Build history of the part. All positions in model axes, mm. Give positions to 0.01 mm unless a question says otherwise; leave off trailing zeros. Order: outer loops, then holes, each group sorted by start corner. A loop starts at its lowest first (then second) coordinate and runs counter-clockwise, first axis right, second up. Notation, with made-up numbers: (83, 82) - (108, 82) arc R31 cw to (108, 118) - close; hole circle Ø10 at (37.5, 5). An arc over 180 degrees is marked (long way). Use a Markdown table: item, result. Add a question column.
(1) Wall check: line 1 (X direction, y = 1.45, z = 47.5); line 2 (X direction, y = 6.85, z = -47.5); line 3 (Z direction, x = -26, y = 7.25) (3 decimals). Give the ranges that are in metal, low to high.
(2) Slice it at B-B (z = 8.5). Write the cut outline in (x, y), then the cut area to 3 significant figures.
(3) Slice it at C-C (y = 3.25). Count the separate pieces of the cut face and the enclosed holes in it, then the cut area to 3 significant figures.
(4) Flat gauge pins, fed straight in: pin 1 (2 mm diameter, centred on x = 72, z = 46.5, fed in from +Y); pin 2 (1.5 mm diameter, centred on x = -44.5, z = -10, fed in from -Y); pin 3 (4 mm diameter, centred on x = 8.5, z = -37.5, fed in from +Y); pin 4 (3 mm diameter, centred on x = -72.28, z = -47.5, fed in from +Y). Where does each tip first touch, or does it go through?
(5) Slice it at A-A (z = -47.5). Write the cut outline in (x, y), then the cut area to 3 significant figures.
from build123d import *

# Parameters (mm, degrees)
BOSS_EXTRUDE1_DEPTH           = 57.5
CUT_EXTRUDE1_DEPTH            = 7
CUT_EXTRUDE4_START            = -7
CUT_EXTRUDE4_DEPTH            = 99.838825225
CBORE_FOR_M3_SHCS1_AT_2_COUNT = 2
CBORE_FOR_M3_SHCS1_AT_2_PITCH = 95
CBORE_FOR_M3_SHCS1_AT_3_COUNT = 2
CBORE_FOR_M3_SHCS1_AT_3_PITCH = 144.569240482
CBORE_FOR_M3_SHCS1_AT_4_COUNT = 2
CBORE_FOR_M3_SHCS1_AT_4_PITCH = 172.989205714
SKETCH14_R                    = 3.25
CUT_EXTRUDE5_DEPTH            = 102.795596501


with BuildPart() as part:
    # Sketch1 → Boss-Extrude1 (new, symmetric)
    with BuildSketch(Plane.XY):
        Polygon((-82.284620241, 0), (82.284620241, 0), (82.284620241, 8), (3.5, 21.891854213), (-3.5, 21.891854213), (-82.284620241, 8), align=None)
    extrude(amount=BOSS_EXTRUDE1_DEPTH, both=True)

    # Sketch2 → Cut-Extrude1 (cut)
    with BuildSketch(Plane(origin=(-3.849265471, 21.830269287, 0), x_dir=(0.9848077530122079, 0.17364817766693139, 0), z_dir=(-0.17364817766693139, 0.9848077530122079, 0))):
        with BuildLine():
            Line((-46.110814579, 26.6), (-36.110814579, 26.6))
            ThreePointArc((-36.110814579, 26.6), (-34.510814579, 25), (-36.110814579, 23.4))
            Line((-36.110814579, 23.4), (-46.110814579, 23.4))
            ThreePointArc((-46.110814579, 23.4), (-47.710814579, 25), (-46.110814579, 26.6))
        make_face()
        with BuildLine():
            Line((-11.110814579, -26.6), (-21.110814579, -26.6))
            ThreePointArc((-21.110814579, -26.6), (-22.710814579, -25), (-21.110814579, -23.4))
            Line((-21.110814579, -23.4), (-11.110814579, -23.4))
            ThreePointArc((-11.110814579, -23.4), (-9.510814579, -25), (-11.110814579, -26.6))
        make_face()
        with BuildLine():
            Line((-11.110814579, 26.6), (-21.110814579, 26.6))
            ThreePointArc((-21.110814579, 26.6), (-22.710814579, 25), (-21.110814579, 23.4))
            Line((-21.110814579, 23.4), (-11.110814579, 23.4))
            ThreePointArc((-11.110814579, 23.4), (-9.510814579, 25), (-11.110814579, 26.6))
        make_face()
        with BuildLine():
            Line((-46.110814579, -26.6), (-36.110814579, -26.6))
            ThreePointArc((-36.110814579, -26.6), (-34.510814579, -25), (-36.110814579, -23.4))
            Line((-36.110814579, -23.4), (-46.110814579, -23.4))
            ThreePointArc((-46.110814579, -23.4), (-47.710814579, -25), (-46.110814579, -26.6))
        make_face()
    cut_extrude1 = extrude(amount=-CUT_EXTRUDE1_DEPTH, mode=Mode.SUBTRACT)

    # Sketch7 → Cut-Extrude4 (cut, through all)
    # profile 1 of 10: a face of its own
    with BuildSketch(Plane(origin=(-3.849265471, 21.830269287, 0), x_dir=(0.9848077530122079, 0.1736481776669313, 0), z_dir=(-0.1736481776669313, 0.9848077530122079, 0)).offset(CUT_EXTRUDE4_START)):
        with BuildLine():
            ThreePointArc((-32.360814579, 22.125), (-30.327882583, 22.967068004), (-29.485814579, 25))
            Line((-29.485814579, 25), (-34.510814579, 25))
            ThreePointArc((-34.510814579, 25), (-34.979443729, 23.86862915), (-36.110814579, 23.4))
            Line((-36.110814579, 23.4), (-41.110814579, 23.4))
            Line((-41.110814579, 23.4), (-41.110814579, 22.125))
            Line((-41.110814579, 22.125), (-32.360814579, 22.125))
        make_face()
    # profile 2 of 10: a face of its own
    with BuildSketch(Plane(origin=(-3.849265471, 21.830269287, 0), x_dir=(0.9848077530122079, 0.1736481776669313, 0), z_dir=(-0.1736481776669313, 0.9848077530122079, 0)).offset(CUT_EXTRUDE4_START)):
        with BuildLine():
            Line((-32.360814579, 27.875), (-49.860814579, 27.875))
            ThreePointArc((-49.860814579, 27.875), (-52.735814579, 25), (-49.860814579, 22.125))
            Line((-49.860814579, 22.125), (-41.110814579, 22.125))
            Line((-41.110814579, 22.125), (-41.110814579, 23.4))
            Line((-41.110814579, 23.4), (-46.110814579, 23.4))
            ThreePointArc((-46.110814579, 23.4), (-47.710814579, 25), (-46.110814579, 26.6))
            Line((-46.110814579, 26.6), (-36.110814579, 26.6))
            ThreePointArc((-36.110814579, 26.6), (-34.979443729, 26.13137085), (-34.510814579, 25))
            Line((-34.510814579, 25), (-29.485814579, 25))
            ThreePointArc((-29.485814579, 25), (-30.327882583, 27.032931996), (-32.360814579, 27.875))
        make_face()
    # profile 3 of 10: a face of its own
    with BuildSketch(Plane(origin=(-3.849265471, 21.830269287, 0), x_dir=(0.9848077530122079, 0.1736481776669313, 0), z_dir=(-0.1736481776669313, 0.9848077530122079, 0)).offset(CUT_EXTRUDE4_START)):
        with BuildLine():
            ThreePointArc((-36.110814579, 23.4), (-34.979443729, 23.86862915), (-34.510814579, 25))
            Line((-34.510814579, 25), (-41.110814579, 25))
            Line((-41.110814579, 25), (-41.110814579, 23.4))
            Line((-41.110814579, 23.4), (-36.110814579, 23.4))
        make_face()
    # profile 4 of 10: a face of its own
    with BuildSketch(Plane(origin=(-3.849265471, 21.830269287, 0), x_dir=(0.9848077530122079, 0.1736481776669313, 0), z_dir=(-0.1736481776669313, 0.9848077530122079, 0)).offset(CUT_EXTRUDE4_START)):
        with BuildLine():
            Line((-41.110814579, 25), (-34.510814579, 25))
            ThreePointArc((-34.510814579, 25), (-34.979443729, 26.13137085), (-36.110814579, 26.6))
            Line((-36.110814579, 26.6), (-46.110814579, 26.6))
            ThreePointArc((-46.110814579, 26.6), (-47.710814579, 25), (-46.110814579, 23.4))
            Line((-46.110814579, 23.4), (-41.110814579, 23.4))
            Line((-41.110814579, 23.4), (-41.110814579, 25))
        make_face()
    # profile 5 of 10: a face of its own
    with BuildSketch(Plane(origin=(-3.849265471, 21.830269287, 0), x_dir=(0.9848077530122079, 0.1736481776669313, 0), z_dir=(-0.1736481776669313, 0.9848077530122079, 0)).offset(CUT_EXTRUDE4_START)):
        with BuildLine():
            ThreePointArc((-24.860814579, 22.125), (-27.735814579, 25), (-24.860814579, 27.875))
            Line((-24.860814579, 27.875), (-7.360814579, 27.875))
            ThreePointArc((-7.360814579, 27.875), (-4.485814579, 25), (-7.360814579, 22.125))
            Line((-7.360814579, 22.125), (-24.860814579, 22.125))
        make_face()
        with BuildLine():
            ThreePointArc((-11.110814579, 26.6), (-9.510814579, 25), (-11.110814579, 23.4))
            Line((-11.110814579, 23.4), (-21.110814579, 23.4))
            ThreePointArc((-21.110814579, 23.4), (-22.710814579, 25), (-21.110814579, 26.6))
            Line((-21.110814579, 26.6), (-11.110814579, 26.6))
        make_face(mode=Mode.SUBTRACT)
    # profile 6 of 10: a face of its own
    with BuildSketch(Plane(origin=(-3.849265471, 21.830269287, 0), x_dir=(0.9848077530122079, 0.1736481776669313, 0), z_dir=(-0.1736481776669313, 0.9848077530122079, 0)).offset(CUT_EXTRUDE4_START)):
        with BuildLine():
            Line((-11.110814579, 23.4), (-21.110814579, 23.4))
            ThreePointArc((-21.110814579, 23.4), (-22.710814579, 25), (-21.110814579, 26.6))
            Line((-21.110814579, 26.6), (-11.110814579, 26.6))
            ThreePointArc((-11.110814579, 26.6), (-9.510814579, 25), (-11.110814579, 23.4))
        make_face()
    # profile 7 of 10: a face of its own
    with BuildSketch(Plane(origin=(-3.849265471, 21.830269287, 0), x_dir=(0.9848077530122079, 0.1736481776669313, 0), z_dir=(-0.1736481776669313, 0.9848077530122079, 0)).offset(CUT_EXTRUDE4_START)):
        with BuildLine():
            ThreePointArc((-32.360814579, -22.125), (-29.485814579, -25), (-32.360814579, -27.875))
            Line((-32.360814579, -27.875), (-49.860814579, -27.875))
            ThreePointArc((-49.860814579, -27.875), (-52.735814579, -25), (-49.860814579, -22.125))
            Line((-49.860814579, -22.125), (-32.360814579, -22.125))
        make_face()
        with BuildLine():
            ThreePointArc((-46.110814579, -26.6), (-47.710814579, -25), (-46.110814579, -23.4))
            Line((-46.110814579, -23.4), (-36.110814579, -23.4))
            ThreePointArc((-36.110814579, -23.4), (-34.510814579, -25), (-36.110814579, -26.6))
            Line((-36.110814579, -26.6), (-46.110814579, -26.6))
        make_face(mode=Mode.SUBTRACT)
    # profile 8 of 10: a face of its own
    with BuildSketch(Plane(origin=(-3.849265471, 21.830269287, 0), x_dir=(0.9848077530122079, 0.1736481776669313, 0), z_dir=(-0.1736481776669313, 0.9848077530122079, 0)).offset(CUT_EXTRUDE4_START)):
        with BuildLine():
            Line((-46.110814579, -23.4), (-36.110814579, -23.4))
            ThreePointArc((-36.110814579, -23.4), (-34.510814579, -25), (-36.110814579, -26.6))
            Line((-36.110814579, -26.6), (-46.110814579, -26.6))
            ThreePointArc((-46.110814579, -26.6), (-47.710814579, -25), (-46.110814579, -23.4))
        make_face()
    # profile 9 of 10: a face of its own
    with BuildSketch(Plane(origin=(-3.849265471, 21.830269287, 0), x_dir=(0.9848077530122079, 0.1736481776669313, 0), z_dir=(-0.1736481776669313, 0.9848077530122079, 0)).offset(CUT_EXTRUDE4_START)):
        with BuildLine():
            Line((-7.360814579, -22.125), (-24.860814579, -22.125))
            ThreePointArc((-24.860814579, -22.125), (-27.735814579, -25), (-24.860814579, -27.875))
            Line((-24.860814579, -27.875), (-7.360814579, -27.875))
            ThreePointArc((-7.360814579, -27.875), (-4.485814579, -25), (-7.360814579, -22.125))
        make_face()
        with BuildLine():
            ThreePointArc((-21.110814579, -26.6), (-22.710814579, -25), (-21.110814579, -23.4))
            Line((-21.110814579, -23.4), (-11.110814579, -23.4))
            ThreePointArc((-11.110814579, -23.4), (-9.510814579, -25), (-11.110814579, -26.6))
            Line((-11.110814579, -26.6), (-21.110814579, -26.6))
        make_face(mode=Mode.SUBTRACT)
    # profile 10 of 10: a face of its own
    with BuildSketch(Plane(origin=(-3.849265471, 21.830269287, 0), x_dir=(0.9848077530122079, 0.1736481776669313, 0), z_dir=(-0.1736481776669313, 0.9848077530122079, 0)).offset(CUT_EXTRUDE4_START)):
        with BuildLine():
            Line((-21.110814579, -23.4), (-11.110814579, -23.4))
            ThreePointArc((-11.110814579, -23.4), (-9.510814579, -25), (-11.110814579, -26.6))
            Line((-11.110814579, -26.6), (-21.110814579, -26.6))
            ThreePointArc((-21.110814579, -26.6), (-22.710814579, -25), (-21.110814579, -23.4))
        make_face()
    cut_extrude4 = extrude(amount=-CUT_EXTRUDE4_DEPTH, mode=Mode.SUBTRACT)

    # Mirror1: Cut-Extrude1, Cut-Extrude4 across plane
    add(cut_extrude1.mirror(Plane(origin=(0, 0, 0), x_dir=(0, 0, 1), z_dir=(1, 0, 0))), mode=Mode.SUBTRACT)
    add(cut_extrude4.mirror(Plane(origin=(0, 0, 0), x_dir=(0, 0, 1), z_dir=(1, 0, 0))), mode=Mode.SUBTRACT)

    # Sketch12 → CBORE for M3 SHCS1 (revolve, cut)
    with BuildSketch(Plane(origin=(72.284620241, 8, -47.5), x_dir=(0, 0, 1), z_dir=(1, 0, 0))):
        Polygon((0, 0), (0, 8), (1.8, 8), (1.8, 3), (3.25, 3), (3.25, 0), align=None)
    cbore_for_m3_shcs1 = revolve(axis=Axis((72.284620241, 14.35, -47.5), (0, -1, 0)), mode=Mode.SUBTRACT)

    # CBORE for M3 SHCS1 at 2: CBORE for M3 SHCS1 ×2
    with Locations(*[(0, 0, i * CBORE_FOR_M3_SHCS1_AT_2_PITCH) for i in range(1, CBORE_FOR_M3_SHCS1_AT_2_COUNT)]):
        add(cbore_for_m3_shcs1, mode=Mode.SUBTRACT)

    # CBORE for M3 SHCS1 at 3: CBORE for M3 SHCS1 ×2
    with Locations(*[(-i * CBORE_FOR_M3_SHCS1_AT_3_PITCH, 0, 0) for i in range(1, CBORE_FOR_M3_SHCS1_AT_3_COUNT)]):
        add(cbore_for_m3_shcs1, mode=Mode.SUBTRACT)

    # CBORE for M3 SHCS1 at 4: CBORE for M3 SHCS1 ×2
    with Locations(*[Vector(-0.8357124936514465, 0, 0.5491672131098877) * (i * CBORE_FOR_M3_SHCS1_AT_4_PITCH) for i in range(1, CBORE_FOR_M3_SHCS1_AT_4_COUNT)]):
        add(cbore_for_m3_shcs1, mode=Mode.SUBTRACT)

    # Sketch14 → Cut-Extrude5 (cut, through all)
    with BuildSketch(Plane(origin=(0, 5, 0), x_dir=(1, 0, 0), z_dir=(0, 1, 0))):
        with Locations(Location((-72.284620241, -47.5, 0), (0, 0, 270))):
            Circle(SKETCH14_R)
        with Locations(Location((-72.284620241, 47.5, 0), (0, 0, 270))):
            Circle(SKETCH14_R)
        with Locations(Location((72.284620241, -47.5, 0), (0, 0, 270))):
            Circle(SKETCH14_R)
        with Locations(Location((72.284620241, 47.5, 0), (0, 0, 270))):
            Circle(SKETCH14_R)
    extrude(amount=CUT_EXTRUDE5_DEPTH, mode=Mode.SUBTRACT)


solid = part.part
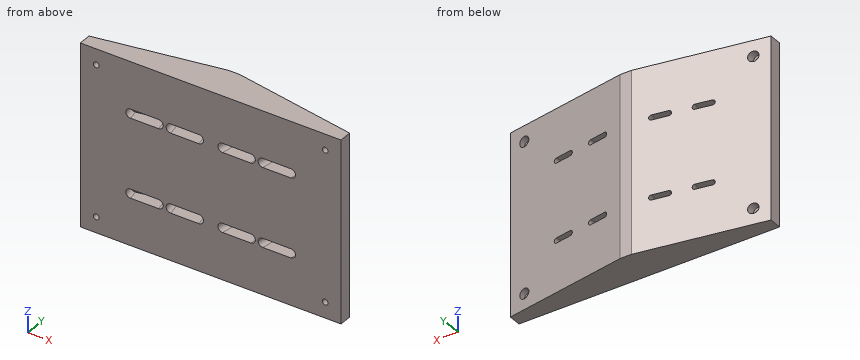
Solution:
| question | item | result |
|---|---|---|
| 1 | line 1 | -82.28 to -74.08, -70.48 to 70.48, 74.08 to 82.28 |
| 1 | line 2 | -82.28 to -75.53, -69.03 to 69.03, 75.53 to 82.28 |
| 1 | line 3 | -57.5 to -27.875, -22.125 to 22.125, 27.875 to 57.5 |
| 2 | outline | (-82.28, 0) - (82.28, 0) - (82.28, 8) - (3.5, 21.89) - (-3.5, 21.89) - (-82.28, 8) - close |
| 2 | area | 2,510 mm2 |
| 3 | separate pieces | 1 |
| 3 | enclosed holes | 12 |
| 3 | area | 17,900 mm2 |
| 4 | pin 1 | y = 5 |
| 4 | pin 2 | y = 0 |
| 4 | pin 3 | y = 21.36 |
| 4 | pin 4 | through |
| 5 | outline | (-82.28, 0) - (-74.08, 0) - (-74.08, 5) - (-75.53, 5) - (-75.53, 9.19) - (-82.28, 8) - close; (-70.48, 0) - (70.48, 0) - (70.48, 5) - (69.03, 5) - (69.03, 10.34) - (3.5, 21.89) - (-3.5, 21.89) - (-69.03, 10.34) - (-69.03, 5) - (-70.48, 5) - close; (74.08, 0) - (82.28, 0) - (82.28, 8) - (75.53, 9.19) - (75.53, 5) - (74.08, 5) - close |
| 5 | area | 2,410 mm2 |
